Model file for the job. Use its own axes, mm. A direction names the side the tool comes from. Round coordinates to 2 decimals unless told otherwise and drop trailing zeros. Loops run counter-clockwise (first coordinate to the right, second up) from the corner with the lowest first, then second, coordinate; pieces in that order, holes last. Notation, with made-up numbers: M -3,76 L 12,76 A24 ccw 12,90 Z; hole C 85,-1.5 d2. An arc over 180 degrees is marked long. Use a Markdown table: item, result. Add a question column.
Q1. Cut at B-B (y = -6). Give the cut face in (x, z).
Q2. Probe line 1 (Y direction, x = 0, z = 1.9); line 2 (X direction, y = -10.5, z = 1.1); line 3 (Y direction, x = -6, z = 1.5). List the from-to ranges inside material, lowest first. Write a range as from..to.
Q3. Cut at A-A (x = 0). Give the cut face in (y, z).
Q4. Cut at C-C (z = 0.9). Give the cut face in (x, y).
Q5. Mould opens along X. For faces 1 (the face through (17, 3, 1)), 2 (the face through (3, 17, 1)), 3 (the face through (-0.17, -6.78, 1.48)) say: +X half, -X half, draft (parallel to the pull), parting line (faces both ways), or undercut.
Q6. Pin check, flat tips, straight feed: pin 1 (1 mm diameter, centred on x = -6.5, z = 2.5, fed in from +Y); pin 2 (1.5 mm diameter, centred on y = -16, z = 1, fed in from -X); pin 3 (1.5 mm diameter, centred on y = -14.5, z = 1.5, fed in from +X). Stop position of each tip, or through.
Q7. Tool access for faces 4 (the face through (-3, 17, 1)), 5 (the face through (3, -17, 1)), 6 (the face through (-17, -3, 1)): list every direction of +Z, -Z, +X, -X, +Y, -Y with a clear straight run to the whole face (end or side of a thin tool).
from build123d import *

# Parameters (mm, degrees)
SKETCH1_R           = 0.8
BOSS_EXTRUDE1_DEPTH = 3
FILLET1_R           = 6
SKETCH2_R           = 2
CUT_EXTRUDE1_DEPTH  = 3


with BuildPart() as part:
    # Sketch1 → Boss-Extrude1 (new body)
    # profile 1 of 2: a face of its own
    with BuildSketch(Plane.XY):
        with BuildLine():
            Line((25, -3), (-25, -3))
            ThreePointArc((-25, -3), (-28, 0), (-25, 3))
            Line((-25, 3), (25, 3))
            ThreePointArc((25, 3), (28, 0), (25, -3))
        make_face()
        with Locations((-6, 0)):
            Circle(SKETCH1_R, mode=Mode.SUBTRACT)
        with Locations((6, 0)):
            Circle(SKETCH1_R, mode=Mode.SUBTRACT)
    # profile 2 of 2: a face of its own
    with BuildSketch(Plane.XY):
        with BuildLine():
            Line((-3, -25), (-3, 25))
            ThreePointArc((-3, 25), (0, 28), (3, 25))
            Line((3, 25), (3, -25))
            ThreePointArc((3, -25), (0, -28), (-3, -25))
        make_face()
        with Locations((0, 6)):
            Circle(SKETCH1_R, mode=Mode.SUBTRACT)
        with Locations((0, -6)):
            Circle(SKETCH1_R, mode=Mode.SUBTRACT)
    extrude(amount=BOSS_EXTRUDE1_DEPTH)

    # Fillet1
    fillet1_edges = [part.edges().sort_by_distance(p)[0] for p in [
        (3, -3, 1.5),
        (-3, -3, 1.5),
        (-3, 3, 1.5),
        (3, 3, 1.5),
    ]]
    fillet(fillet1_edges, radius=FILLET1_R)

    # Sketch2 → Cut-Extrude1 (cut)
    with BuildSketch(Plane.XY.offset(3)):
        Circle(SKETCH2_R)
    extrude(amount=-CUT_EXTRUDE1_DEPTH, mode=Mode.SUBTRACT)


solid = part.part
Checked values:
| question | item | result |
|---|---|---|
| 1 | outline | M -3.8,0 L -0.8,0 L -0.8,3 L -3.8,3 Z; M 0.8,0 L 3.8,0 L 3.8,3 L 0.8,3 Z |
| 2 | line 1 | y = -28..-6.8, -5.2..-2, 2..5.2, 6.8..28 |
| 2 | line 2 | x = -3..3 |
| 2 | line 3 | y = -3.8..-0.8, 0.8..3.8 |
| 3 | outline | M -28,0 L -6.8,0 L -6.8,3 L -28,3 Z; M -5.2,0 L -2,0 L -2,3 L -5.2,3 Z; M 2,0 L 5.2,0 L 5.2,3 L 2,3 Z; M 6.8,0 L 28,0 L 28,3 L 6.8,3 Z |
| 4 | outline | M -25,-3 L -9,-3 A6 cw -3,-9 L -3,-25 A3 ccw 3,-25 L 3,-9 A6 cw 9,-3 L 25,-3 A3 ccw 25,3 L 9,3 A6 cw 3,9 L 3,25 A3 ccw -3,25 L -3,9 A6 cw -9,3 L -25,3 A3 ccw Z; hole C -6,0 d1.6; hole C 0,0 d4; hole C 0,-6 d1.6; hole C 0,6 d1.6; hole C 6,0 d1.6 |
| 5 | face 1 | draft |
| 5 | face 2 | +X half |
| 5 | face 3 | undercut |
| 6 | pin 1 | stops at y = 3.8 |
| 6 | pin 2 | stops at x = -3 |
| 6 | pin 3 | stops at x = 3 |
| 7 | face 4 | +Z, -Z, -X, +Y |
| 7 | face 5 | +Z, -Z, +X, -Y |
| 7 | face 6 | +Z, -Z, -X, -Y |
